The listing builds one solid part. Answer for the finished solid, in the listing's coordinates (mm). Face numbers are marked on the shaded views. A direction names the side the tool comes from. Coordinates: 2 decimals unless noted, no trailing zeros. Loops run counter-clockwise (first coordinate to the right, second up) from the corner with the lowest first, then second, coordinate; pieces in that order, holes last. Notation, with made-up numbers: M 5,-29.5 L 37,-29.5 A20 ccw 37,-25.5 Z; hole C -26,65 d9. An arc over 180 degrees is marked long. Answer as a JSON object with one key per item and string values. Group by question number.
1. A cutting plane is placed at C-C on x = -4.5. Give the vertices of the cut face in (y, z), and give its area (3 significant figures).
2. A cutting plane is placed at A-A on x = 0. Give the vertices of the cut face in (y, z).
3. A cutting plane is placed at B-B on y = 3. Give the vertices of the cut face in (x, z).
4. A cutting plane is placed at D-D on y = 15. Give the vertices of the cut face in (x, z).
5. For the marked faces 1, 2 and 3, determine the directions among +Z, -Z, +X, -X, +Y, -Y from which every point of the face is accessible in a straight line to the end or side of a thin tool.
6. Straight lines are drawn through the part: L1, parallel to Y at x = 0, z = 3; L2, parallel to Y at x = 0, z = 1.5; L3, parallel to X at y = -4, z = 3.5. For each, find the intervals that lie inside material, in ascending order.
7. Determine the mould class of the marked faces 4, 5 and 6 for opening direction X: released by +X, released by -X, zero draft, split by the parting line, or undercut.
8. Given pin 1 (0.6 mm diameter, centred on x = 4, y = 0, fed in from +Z); pin 2 (3.5 mm diameter, centred on x = -9.5, y = 0.5, fed in from +Z); pin 3 (1.8 mm diameter, centred on x = -9, z = 5.5, fed in from +Y); pin 4 (3 mm diameter, centred on x = 0, y = 15, fed in from -Z), each flat-ended and moving along its own axis, determine where each tip first touches the part or whether it passes through.
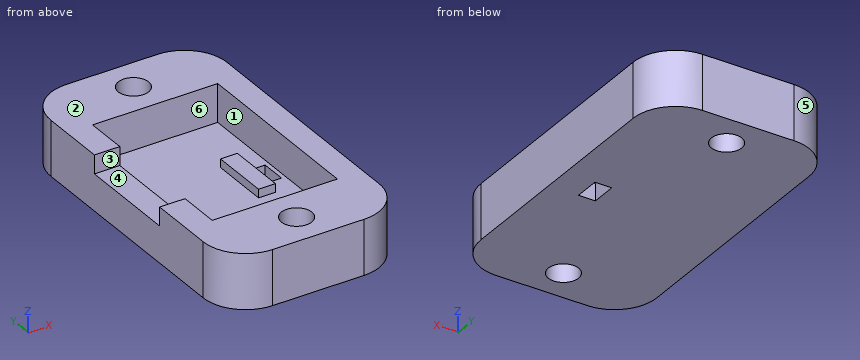
from build123d import *

# Parameters (mm, degrees)
F0_R     = 1.8
F1_DEPTH = 6.5
F2_DEPTH = 2
F3_DEPTH = 3
F0_W     = 3
F0_H     = 12
F4_DEPTH = 4.3
F5_R     = 5


with BuildPart() as f1:
    # F0 (on Top) → F1 (new body)
    with BuildSketch(Plane.XY):
        Polygon((-7.4, 6), (-7.4, 11), (7.4, 11), (7.4, -11), (-7.4, -11), (-7.4, -6), (-10.4, -6), (-10.4, -19), (10.4, -19), (10.4, 19), (-10.4, 19), (-10.4, 6), align=None)
        with Locations((0, -15)):
            Circle(F0_R, mode=Mode.SUBTRACT)
        with Locations((0, 15)):
            Circle(F0_R, mode=Mode.SUBTRACT)
    extrude(amount=F1_DEPTH)

    # F0 (on Top) → F2 (join)
    with BuildSketch(Plane.XY):
        Polygon((7.4, 11), (-7.4, 11), (-7.4, 6), (-7.4, -6), (-7.4, -11), (7.4, -11), align=None)
        Polygon((2.9, -3.5), (2.9, 3.5), (4.9, 3.5), (4.9, 1.5), (6.9, 1.5), (6.9, -1.5), (4.9, -1.5), (4.9, -3.5), align=None, mode=Mode.SUBTRACT)
    extrude(amount=F2_DEPTH)

    # F0 (on Top) → F3 (join)
    with BuildSketch(Plane.XY):
        Polygon((4.9, 3.5), (2.9, 3.5), (2.9, -3.5), (4.9, -3.5), (4.9, -1.5), (4.9, 1.5), align=None)
    extrude(amount=F3_DEPTH)

    # F0 (on Top) → F4 (join)
    with BuildSketch(Plane.XY):
        with Locations((-8.9, 0)):
            Rectangle(F0_W, F0_H)
    extrude(amount=F4_DEPTH)

    # F5
    f5_edges = [f1.edges().sort_by_distance(p)[0] for p in [
        (-10.4, 19, 3.25),
        (10.4, 19, 3.25),
        (-10.4, -19, 3.25),
        (10.4, -19, 3.25),
    ]]
    fillet(f5_edges, radius=F5_R)


solid = f1.part
From the geometry:
{
 "1": {"outline": "M -19,0 L 19,0 L 19,6.5 L 11,6.5 L 11,2 L -11,2 L -11,6.5 L -19,6.5 Z", "area": "148 mm²"},
 "2": {"outline": "M -19,0 L -16.8,0 L -16.8,6.5 L -19,6.5 Z; M -13.2,0 L 13.2,0 L 13.2,6.5 L 11,6.5 L 11,2 L -11,2 L -11,6.5 L -13.2,6.5 Z; M 16.8,0 L 19,0 L 19,6.5 L 16.8,6.5 Z"},
 "3": {"outline": "M -10.4,0 L 10.4,0 L 10.4,6.5 L 7.4,6.5 L 7.4,2 L 4.9,2 L 4.9,3 L 2.9,3 L 2.9,2 L -7.4,2 L -7.4,4.3 L -10.4,4.3 Z"},
 "4": {"outline": "M -10.3,0 L -1.8,0 L -1.8,6.5 L -10.3,6.5 Z; M 1.8,0 L 10.3,0 L 10.3,6.5 L 1.8,6.5 Z"},
 "5": {"face 1": "+Z", "face 2": "+Z, +X, -X, +Y, -Y", "face 3": "+Z, -X"},
 "6": {"L1": "y = -19 to -16.8, -13.2 to -11, 11 to 13.2, 16.8 to 19", "L2": "y = -19 to -16.8, -13.2 to 13.2, 16.8 to 19", "L3": "x = -10.4 to -7.4, 7.4 to 10.4"},
 "7": {"face 4": "zero draft", "face 5": "released by -X", "face 6": "undercut"},
 "8": {"pin 1": "stops at z = 3", "pin 2": "stops at z = 4.3", "pin 3": "stops at y = 18.21", "pin 4": "passes through"}
}
